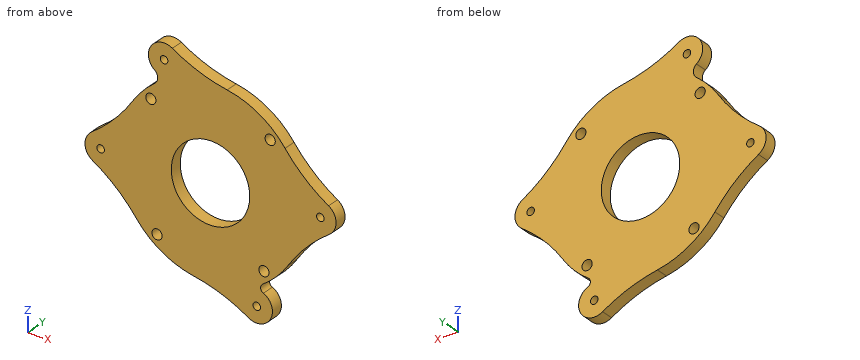
from build123d import *

# Parameters (mm, degrees)
F0_R     = 3.25
F0_R_2   = 2.4
F0_R_3   = 25
F1_DEPTH = 8


with BuildPart() as f1:
    # F0 (on Front) → F1 (new body)
    with BuildSketch(Plane.XZ):
        with BuildLine():
            ThreePointArc((-35.636863, 55.482015), (-33.663679, 51.486611), (-35.661818, 47.503628))
            ThreePointArc((-35.661818, 47.503628), (-43.197676, 40.771569), (-49.483404, 32.859591))
            ThreePointArc((-49.483404, 32.859591), (-61.316735, 18.237762), (-75.678931, 6.090625))
            ThreePointArc((-75.678931, 6.090625), (-79.963365, -2.420787), (-75.171905, -10.657439))
            ThreePointArc((-75.171905, -10.657439), (-60.101207, -21.913533), (-47.405043, -35.792763))
            ThreePointArc((-47.405043, -35.792763), (-31.204449, -50.54347), (-10.758408, -58.417606))
            ThreePointArc((-10.758408, -58.417606), (7.338328, -63.549248), (24.153913, -71.979058))
            ThreePointArc((24.153913, -71.979058), (38.248014, -68.265692), (33.665686, -54.429687))
            ThreePointArc((33.665686, -54.429687), (31.938042, -51.947575), (33.24924, -49.222435))
            ThreePointArc((33.24924, -49.222435), (42.12576, -41.878161), (49.41758, -32.958501))
            ThreePointArc((49.41758, -32.958501), (61.280134, -18.36037), (75.666598, -6.241984))
            ThreePointArc((75.666598, -6.241984), (79.968047, 2.260842), (75.193072, 10.507061))
            ThreePointArc((75.193072, 10.507061), (60.144918, 21.793276), (47.47654, 35.697873))
            ThreePointArc((47.47654, 35.697873), (31.204449, 50.54347), (10.641541, 58.439008))
            ThreePointArc((10.641541, 58.439008), (-7.465423, 63.534443), (-24.297835, 71.930602))
            ThreePointArc((-24.297835, 71.930602), (-37.816535, 69.117238), (-35.636863, 55.482015))
        make_face()
        with Locations((-34.077461, -41.242898)):
            Circle(F0_R, mode=Mode.SUBTRACT)
        with Locations((-69.967945, -2.118189)):
            Circle(F0_R_2, mode=Mode.SUBTRACT)
        with Locations((29.456325, -63.50059)):
            Circle(F0_R_2, mode=Mode.SUBTRACT)
        with Locations((34.022539, -41.288217)):
            Circle(F0_R, mode=Mode.SUBTRACT)
        Circle(F0_R_3, mode=Mode.SUBTRACT)
        with Locations((-38, 37.65966)):
            Circle(F0_R, mode=Mode.SUBTRACT)
        with Locations((-29.583278, 63.441545)):
            Circle(F0_R_2, mode=Mode.SUBTRACT)
        with Locations((69.972041, 1.978236)):
            Circle(F0_R_2, mode=Mode.SUBTRACT)
        with Locations((38, 37.65966)):
            Circle(F0_R, mode=Mode.SUBTRACT)
    extrude(amount=F1_DEPTH)


solid = f1.part
Verification items for the finished model (mm, model axes). Coordinates: 2 decimals unless noted, no trailing zeros. Write each loop counter-clockwise with the first axis right and the second up, starting at its lowest first coordinate (ties: lowest second). Pieces come first, ordered by that corner, then holes. Notation, with made-up numbers: M -17.75,73 L 24.25,73 A18 ccw 24.25,78 Z; hole C 2.25,37.5 d4. An arc over 180 degrees is marked long. Use a Markdown table: item, result.
Q1. Sectioned sample at A-A, the plane x = 7.5. Record the boundary of the cut face in (y, z).
Reply:
| item | result |
|---|---|
| outline | M -8,-63.61 L 0,-63.61 L 0,-23.85 L -8,-23.85 Z; M -8,23.85 L 0,23.85 L 0,59.06 L -8,59.06 Z |
Q2. Thickness scan on line 1 (X direction, y = -6.5, z = 0.5) (3 decimals); line 2 (X direction, y = -7.25, z = 20); line 3 (X direction, y = -4.75, z = 36.5). Record the ranges inside material, lowest first.
Reply:
| item | result |
|---|---|
| line 1 | x = -79.619 to -24.995, 24.995 to 68.081, 71.863 to 79.862 |
| line 2 | x = -59.63 to -15, 15 to 62.17 |
| line 3 | x = -46.86 to -41.04, -34.96 to 34.96, 41.04 to 46.86 |
Q3. Sectioned sample at B-B, the plane y = -6. Count the separate pieces of the cut face and the enclosed holes in it, plus the area to 3 significant figures.
Reply:
| item | result |
|---|---|
| separate pieces | 1 |
| enclosed holes | 9 |
| area | 11,100 mm² |
Q4. Sectioned sample at D-D, the plane z = 45.5. Record the boundary of the cut face in (x, y).
Reply:
| item | result |
|---|---|
| outline | M -38.19,-8 L 38.19,-8 L 38.19,0 L -38.19,0 Z |
Q5. Sectioned sample at C-C, the plane x = -21. Record the boundary of the cut face in (y, z).
Reply:
| item | result |
|---|---|
| outline | M -8,-55.56 L 0,-55.56 L 0,-13.56 L -8,-13.56 Z; M -8,13.56 L 0,13.56 L 0,69.96 L -8,69.96 Z |
Q6. Go/stop test with flat-tipped pins: P1, Ø3, axis at x = -2.5, y = -5, coming from the -Z side; P2, Ø4, axis at x = -29.58, z = 63.44, coming from the +Y side; P3, Ø3, axis at x = -19.5, y = -3, coming from the -Z side; P4, Ø1, axis at y = -3.5, z = 19, coming from the +X side. Record where each tip stops, or that it passes through.
Reply:
| item | result |
|---|---|
| P1 | stops at z = -60.73 |
| P2 | passes through |
| P3 | stops at z = -56.61 |
| P4 | stops at x = 63.96 |
